from build123d import *

# Parameters (mm, degrees)
F0_W      = 152
F0_H      = 31.4
F1_DEPTH  = 9
F2_R      = 2
F3_W      = 3
F3_H      = 26.9515514374
F4_DEPTH  = 8.7
F5_DEPTH  = 2
F6_DEPTH  = 2
F7_W      = 1.5
F7_H      = 27.4
F8_DEPTH  = 1.5
F9_W      = 1.5
F9_H      = 27.4
F10_DEPTH = 1.5
F11_D     = 12
F11_DEPTH = 10
F11_TIP   = 3.6051637142


with BuildPart() as f1:
    # F0 (on Front) → F1 (new body)
    with BuildSketch(Plane.XZ):
        Rectangle(F0_W, F0_H)
    extrude(amount=F1_DEPTH)

    # F2
    f2_edges = [f1.edges().sort_by_distance(p)[0] for p in [
        (76, -4.5, 15.7),
        (76, -4.5, -15.7),
        (-76, -4.5, -15.7),
        (-76, -4.5, 15.7),
    ]]
    fillet(f2_edges, radius=F2_R)

    # F3 (on face) → F4 (join)
    with BuildSketch(Plane.XZ.offset(9)):
        with Locations((-74, 0)):
            Rectangle(F3_W, F3_H)
        with Locations((74, -0.0208395504)):
            Rectangle(F3_W, F3_H)
    extrude(amount=F4_DEPTH)

    # F5 (add): a face of the model
    f5_faces = [f1.faces().sort_by_distance(p)[0] for p in [
        (-75.5, -13.35, 0),
    ]]
    extrude(f5_faces, amount=F5_DEPTH)

    # F6 (add): a face of the model
    f6_faces = [f1.faces().sort_by_distance(p)[0] for p in [
        (75.5, -13.35, -0.0208395504),
    ]]
    extrude(f6_faces, amount=F6_DEPTH)

    # F7 (on face) → F8 (join)
    with BuildSketch(Plane(origin=(-76, 0, 0), x_dir=(0, -1, 0), z_dir=(-1, 0, 0))):
        with Locations((0.75, 0)):
            Rectangle(F7_W, F7_H)
    extrude(amount=F8_DEPTH)

    # F9 (on face) → F10 (join)
    with BuildSketch(Plane.YZ.offset(76)):
        with Locations((-0.75, 0)):
            Rectangle(F9_W, F9_H)
    extrude(amount=F10_DEPTH)

    # F11
    with Locations(Plane(origin=(0, 0, 0), x_dir=(1, 0, 0), z_dir=(0, 1, 0))):
        with Locations((-50.7, 0), (-25.3, 0), (25.3, 0), (0, 0), (50.7, 0)):
            Hole(F11_D / 2, depth=F11_DEPTH)
            with Locations((0, 0, -(F11_DEPTH + F11_TIP / 2))):  # 118° drill point
                Cone(0, F11_D / 2, F11_TIP, mode=Mode.SUBTRACT)


solid = f1.part
Read the model definition and answer for the solid it produces. Units are mm, in the model's axes. Round coordinates to 2 decimals unless told otherwise and drop trailing zeros. Write each loop counter-clockwise with the first axis right and the second up, starting at its lowest first coordinate (ties: lowest second). Pieces come first, ordered by that corner, then holes.
1. The part is cut by section C-C, the plane y = -4.5. Determine the outline of the cut face in (x, z).
2. Straight lines are drawn through the part: L1, parallel to Z at x = 50.7, y = -5.5; L2, parallel to X at y = -10.75, z = -7; L3, parallel to X at y = -7.25, z = -2. For each, find the intervals that lie inside material, in ascending order.
3. Given pin 1 Ø1.5 at (x, y) = (-74, -12) entering from +Z; pin 2 Ø6 at (x, z) = (-26.5, 10.5) entering from +Y; pin 3 Ø2.5 at (x, y) = (75.5, -15.5) entering from -Z; pin 4 Ø4 at (x, z) = (-43.5, 9.5) entering from -Y, each flat-ended and moving along its own axis, determine where each tip first touches the part or whether it passes through.
4. The part is cut by section B-B, the plane y = -15. Determine the outline of the cut face in (x, z).
5. The part is cut by section D-D, the plane z = 0. State how many separate pieces and enclosed holes the cut face has, then the cut area to 4 significant figures.
6. The part is cut by section A-A, the plane x = 0. Determine the outline of the cut face in (y, z).
7. Determine the mould class of faces 1 (the face through (77.5, -13, 0)), 2 (the face through (72.5, -13, 0)), 3 (the face through (-75, -13, 13.476)), 4 (the face through (-76, -5, 0)) for opening direction X: pulls with the +X half, pulls with the -X half, needs draft (parallel to the pull), parting line crosses it, or undercut.
Values:
1. outline: (-76, -13.7) arc R2 ccw to (-74, -15.7) - (74, -15.7) arc R2 ccw to (76, -13.7) - (76, 13.7) arc R2 ccw to (74, 15.7) - (-74, 15.7) arc R2 ccw to (-76, 13.7) - close; hole circle Ø12 at (-50.7, 0); hole circle Ø12 at (-25.3, 0); hole circle Ø12 at (0, 0); hole circle Ø12 at (25.3, 0); hole circle Ø12 at (50.7, 0)
2. L1: z = -15.7 to -6, 6 to 15.7
2. L2: x = -77.5 to -72.5, 72.5 to 77.5
2. L3: x = -76 to -56.36, -45.04 to -30.96, -19.64 to -5.66, 5.66 to 19.64, 30.96 to 45.04, 56.36 to 76
3. pin 1: stops at z = 13.48
3. pin 2: stops at y = 0
3. pin 3: stops at z = -13.5
3. pin 4: stops at y = -9
4. outline: (-77.5, -13.48) - (-72.5, -13.48) - (-72.5, 13.48) - (-77.5, 13.48) - close; (72.5, -13.5) - (77.5, -13.5) - (77.5, 13.45) - (72.5, 13.45) - close
5. separate pieces: 6
5. enclosed holes: 0
5. area: 919.5 mm2
6. outline: (-9, -15.7) - (0, -15.7) - (0, -6) - (-9, -6) - close; (-9, 6) - (0, 6) - (0, 15.7) - (-9, 15.7) - close
7. face 1: pulls with the +X half
7. face 2: undercut
7. face 3: needs draft
7. face 4: pulls with the -X half
